The model under review builds one solid part; all positions refer to its coordinate system, in mm. A direction names the side the tool comes from. Coordinates: 2 decimals unless noted, no trailing zeros. Order: outer loops, then holes, each group sorted by start corner. A loop starts at its lowest first (then second) coordinate and runs counter-clockwise, first axis right, second up. Notation, with made-up numbers: M 54.5,-33.5 L 70.5,-33.5 A34 ccw 70.5,-3.5 Z; hole C 44,44 d7. An arc over 180 degrees is marked long. Answer as CSV lines item,"result". Start each with the question number.
Q1. Consider section C-C on x = 0. Write out the cut boundary in (y, z).
Q2. Consider section A-A on z = 0. Write out the cut boundary in (x, y), and give its area (3 significant figures).
Q3. For P1, Ø6.5, axis at x = 30, z = -12.5, coming from the +Y side; P2, Ø6, axis at y = 1.5, z = 11.5, coming from the +X side; P3, Ø1.5, axis at x = 27.5, y = 5, coming from the -Z side, all flat-tipped, find the tip position at first contact; note any pin that passes through.
Q4. The part is to be moulded in two halves that separate along Y. For faces 5 (the face through (15, 12, 24)), 6 (the face through (8.778, 8.307, 18.025)), 7 (the face through (8.69, 10.02, -15.19)), say which applies: +Y half, -Y half, draft (parallel to the pull), parting line (faces both ways), or undercut.
Q5. Machinability: for faces 1 (the face through (27.22, 3.43, -4.4)), 2 (the face through (11.405, 5.555, -14.914)), 3 (the face through (19.769, 9.465, 19.754)), 4 (the face through (-25, 2, -16)), which of the approach directions +Z, -Z, +X, -X, +Y, -Y give a long, thin tool a straight path to every point of the face, cutting with its end or side? Answer none if there is none.
Q6. Consider section B-B on y = 10.75. Write out the cut boundary in (x, z), and give its area (3 significant figures).
Q7. Consider section D-D on x = 31. Write out the cut boundary in (y, z), and give its area (3 significant figures).
Q8. Wall thickness on L1, parallel to X at y = 3.5, z = -13.75; L2, parallel to Z at x = 0, y = 3.7; L3, parallel to Z at x = 0, y = 1.35: over which ranges is each line inside the solid? List them lowest first. Write a range as [from, to].
from build123d import *

# Parameters (mm, degrees)
SKETCH1_R                = 37.5
SKETCH1_R_2              = 2.3
BOSS_EXTRUDE1_DEPTH      = 2
SKETCH2_R                = 37.5
SKETCH2_R_2              = 4.5
BOSS_EXTRUDE2_DEPTH      = 5
BOSS_EXTRUDE3_DEPTH      = 5
SKETCH4_R                = 17.5
CUT_EXTRUDE1_DEPTH       = 7
CUT_EXTRUDE2_DEPTH       = 7
CUT_EXTRUDE2_DEPTH_BACK  = 2.5
CUT_EXTRUDE4_DEPTH       = 3
CUT_EXTRUDE4_DEPTH_BACK  = 2.5
SKETCH10_R               = 1.65
CUT_EXTRUDE7_DEPTH       = 20
SKETCH9_R                = 1.65
CUT_EXTRUDE6_DEPTH       = 20
CUT_EXTRUDE8_DEPTH       = 4
CUT_EXTRUDE9_DEPTH       = 10
CUT_EXTRUDE9_DEPTH_BACK  = 2.5
SKETCH16_R               = 1.65
CUT_EXTRUDE10_DEPTH      = 20
CUT_EXTRUDE11_DEPTH      = 10
CUT_EXTRUDE11_DEPTH_BACK = 2.5
SKETCH18_R               = 1.65
CUT_EXTRUDE12_DEPTH      = 20
FILLET1_R                = 2


with BuildPart() as part:
    # Sketch1 → Boss-Extrude1 (new body)
    with BuildSketch(Plane(origin=(0, 0, 0), x_dir=(1, 0, 0), z_dir=(0, 1, 0))):
        Circle(SKETCH1_R)
        with Locations((0, 27.5)):
            Circle(SKETCH1_R_2, mode=Mode.SUBTRACT)
        with Locations((23.815698604, 13.75)):
            Circle(SKETCH1_R_2, mode=Mode.SUBTRACT)
        with Locations((23.815698604, -13.75)):
            Circle(SKETCH1_R_2, mode=Mode.SUBTRACT)
        with Locations((0, -27.5)):
            Circle(SKETCH1_R_2, mode=Mode.SUBTRACT)
        with Locations((-23.815698604, -13.75)):
            Circle(SKETCH1_R_2, mode=Mode.SUBTRACT)
        with Locations((-23.815698604, 13.75)):
            Circle(SKETCH1_R_2, mode=Mode.SUBTRACT)
    extrude(amount=BOSS_EXTRUDE1_DEPTH)

    # Sketch2 → Boss-Extrude2 (add)
    with BuildSketch(Plane(origin=(0, 2, 0), x_dir=(1, 0, 0), z_dir=(0, 1, 0))):
        Circle(SKETCH2_R)
        with Locations((-23.815698604, 13.75)):
            Circle(SKETCH2_R_2, mode=Mode.SUBTRACT)
        with Locations((-23.815698604, -13.75)):
            Circle(SKETCH2_R_2, mode=Mode.SUBTRACT)
        with Locations((0, -27.5)):
            Circle(SKETCH2_R_2, mode=Mode.SUBTRACT)
        with Locations((23.815698604, -13.75)):
            Circle(SKETCH2_R_2, mode=Mode.SUBTRACT)
        with Locations((23.815698604, 13.75)):
            Circle(SKETCH2_R_2, mode=Mode.SUBTRACT)
        with Locations((0, 27.5)):
            Circle(SKETCH2_R_2, mode=Mode.SUBTRACT)
    extrude(amount=BOSS_EXTRUDE2_DEPTH)

    # Sketch3 → Boss-Extrude3 (add)
    with BuildSketch(Plane(origin=(0, 7, 0), x_dir=(1, 0, 0), z_dir=(0, 1, 0))):
        with BuildLine():
            ThreePointArc((-16.901898546, -4.536058371), (-17.499998615, -0.006962688), (-16.905502698, 4.52260749))
            Line((-16.905502698, 4.52260749), (-36.226077211, 9.691301765))
            ThreePointArc((-36.226077211, 9.691301765), (-37.499997032, -0.014920046), (-36.218354027, -9.720125081))
            Line((-36.218354027, -9.720125081), (-16.901898546, -4.536058371))
        make_face()
        with BuildLine():
            ThreePointArc((-9.720125081, 36.218354027), (-18.762919655, 32.468490048), (-26.527052262, 26.50595213))
            Line((-26.527052262, 26.50595213), (-12.810223172, 12.800033673))
            Line((-12.810223172, 12.800033673), (-4.698199739, 17.506056765))
            Line((-4.698199739, 17.506056765), (-9.720125081, 36.218354027))
        make_face()
        with BuildLine():
            ThreePointArc((16.901898546, 4.536058371), (17.499998615, 0.006962688), (16.905502698, -4.52260749))
            Line((16.905502698, -4.52260749), (36.226077211, -9.691301765))
            ThreePointArc((36.226077211, -9.691301765), (37.499997032, 0.014920046), (36.218354027, 9.720125081))
            Line((36.218354027, 9.720125081), (16.901898546, 4.536058371))
        make_face()
        with BuildLine():
            Line((-12.805791077, -12.81598516), (-26.50595213, -26.527052262))
            ThreePointArc((-26.50595213, -26.527052262), (-18.737077377, -32.483410095), (-9.691301765, -36.226077211))
            Line((-9.691301765, -36.226077211), (-4.682147808, -17.501864262))
            Line((-4.682147808, -17.501864262), (-12.805791077, -12.81598516))
        make_face()
        with BuildLine():
            Line((4.680172315, 17.49447987), (12.811230656, 12.82142907))
            Line((12.811230656, 12.82142907), (26.50595213, 26.527052262))
            ThreePointArc((26.50595213, 26.527052262), (18.737077377, 32.483410095), (9.691301765, 36.226077211))
            Line((9.691301765, 36.226077211), (4.680172315, 17.49447987))
        make_face()
        with BuildLine():
            Line((12.819708432, -12.809511387), (4.694715176, -17.493072864))
            Line((4.694715176, -17.493072864), (9.720125081, -36.218354027))
            ThreePointArc((9.720125081, -36.218354027), (18.762919655, -32.468490048), (26.527052262, -26.50595213))
            Line((26.527052262, -26.50595213), (12.819708432, -12.809511387))
        make_face()
    extrude(amount=BOSS_EXTRUDE3_DEPTH)

    # Sketch4 → Cut-Extrude1 (cut)
    with BuildSketch(Plane(origin=(0, 7, 0), x_dir=(1, 0, 0), z_dir=(0, 1, 0))):
        Circle(SKETCH4_R)
    extrude(amount=-CUT_EXTRUDE1_DEPTH, mode=Mode.SUBTRACT)

    # Sketch5 → Cut-Extrude2 (cut, two sides)
    with BuildSketch(Plane(origin=(-8.743969443, 0, 15.158924711), x_dir=(-0.866224269, 0, -0.499655397), z_dir=(0.499655397, 0, -0.866224269))) as cut_extrude2_sk:
        with BuildLine():
            Line((1.5, 7), (3.290896534, 7))
            Line((3.290896534, 7), (1.645448267, 9.85))
            Line((1.645448267, 9.85), (-1.645448267, 9.85))
            Line((-1.645448267, 9.85), (-3.290896534, 7))
            Line((-3.290896534, 7), (-1.5, 7))
            ThreePointArc((-1.5, 7), (0, 8.5), (1.5, 7))
        make_face()
        with BuildLine():
            Line((1.645448267, 4.15), (3.290896534, 7))
            Line((3.290896534, 7), (1.5, 7))
            ThreePointArc((1.5, 7), (0, 5.5), (-1.5, 7))
            Line((-1.5, 7), (-3.290896534, 7))
            Line((-3.290896534, 7), (-1.645448267, 4.15))
            Line((-1.645448267, 4.15), (1.645448267, 4.15))
        make_face()
        with BuildLine():
            ThreePointArc((-1.5, 7), (0, 5.5), (1.5, 7))
            Line((1.5, 7), (0, 7))
            Line((0, 7), (-1.5, 7))
        make_face()
        with BuildLine():
            Line((0, 7), (1.5, 7))
            ThreePointArc((1.5, 7), (0, 8.5), (-1.5, 7))
            Line((-1.5, 7), (0, 7))
        make_face()
    extrude(amount=CUT_EXTRUDE2_DEPTH, mode=Mode.SUBTRACT)
    extrude(cut_extrude2_sk.sketch, amount=-CUT_EXTRUDE2_DEPTH_BACK, mode=Mode.SUBTRACT)

    # Sketch7 → Cut-Extrude4 (cut, two sides)
    with BuildSketch(Plane(origin=(8.739633736, 0, 15.161424807), x_dir=(-0.866367132, 0, 0.499407642), z_dir=(-0.499407642, 0, -0.866367132))) as cut_extrude4_sk:
        Polygon((0, 7), (3.270607136, 7), (1.625158868, 9.85), (-1.665737666, 9.85), (-3.311185933, 7), (-0.020289399, 7), align=None)
        Polygon((1.625158868, 4.15), (3.270607136, 7), (0, 7), (-0.020289399, 7), (-3.311185933, 7), (-1.665737666, 4.15), align=None)
    extrude(amount=CUT_EXTRUDE4_DEPTH, mode=Mode.SUBTRACT)
    extrude(cut_extrude4_sk.sketch, amount=-CUT_EXTRUDE4_DEPTH_BACK, mode=Mode.SUBTRACT)

    # Sketch10 → Cut-Extrude7 (cut)
    with BuildSketch(Plane(origin=(8.739633736, 0, 15.161424807), x_dir=(-0.866367132, 0, 0.499407642), z_dir=(-0.499407642, 0, -0.866367132))):
        with Locations((-0.020289399, 7)):
            Circle(SKETCH10_R)
    extrude(amount=-CUT_EXTRUDE7_DEPTH, mode=Mode.SUBTRACT)

    # Sketch9 → Cut-Extrude6 (cut)
    with BuildSketch(Plane(origin=(-9.993107934, 0, 17.324485384), x_dir=(-0.866224269, 0, -0.499655397), z_dir=(0.499655397, 0, -0.866224269))):
        with Locations((0, 6.9)):
            Circle(SKETCH9_R)
    extrude(amount=-CUT_EXTRUDE6_DEPTH, mode=Mode.SUBTRACT)

    # Sketch14 → Cut-Extrude8 (cut)
    with BuildSketch(Plane.XZ):
        with BuildLine():
            Line((17.5, 0), (37.5, 0))
            ThreePointArc((37.5, 0), (37.416199333, 2.505599224), (37.165171868, 5))
            Line((37.165171868, 5), (16.770509831, 5))
            ThreePointArc((16.770509831, 5), (17.316667145, 2.526467688), (17.5, 0))
        make_face()
        with BuildLine():
            Line((16.770509831, -5), (37.165171868, -5))
            ThreePointArc((37.165171868, -5), (37.416199333, -2.505599224), (37.5, 0))
            Line((37.5, 0), (17.5, 0))
            ThreePointArc((17.5, 0), (17.316667145, -2.526467688), (16.770509831, -5))
        make_face()
    extrude(amount=-CUT_EXTRUDE8_DEPTH, mode=Mode.SUBTRACT)

    # Sketch15 → Cut-Extrude9 (cut, two sides)
    with BuildSketch(Plane(origin=(-8.781531952, 0, -15.137195796), x_dir=(0.864982617, 0, -0.501801826), z_dir=(0.501801826, 0, 0.864982617))) as cut_extrude9_sk:
        with BuildLine():
            Line((0, 7), (1.5, 7))
            ThreePointArc((1.5, 7), (0, 8.5), (-1.5, 7))
            Line((-1.5, 7), (0, 7))
        make_face()
        with BuildLine():
            ThreePointArc((-1.5, 7), (0, 5.5), (1.5, 7))
            Line((1.5, 7), (0, 7))
            Line((0, 7), (-1.5, 7))
        make_face()
        with BuildLine():
            Line((1.645448267, 4.15), (3.290896534, 7))
            Line((3.290896534, 7), (1.5, 7))
            ThreePointArc((1.5, 7), (0, 5.5), (-1.5, 7))
            Line((-1.5, 7), (-3.290896534, 7))
            Line((-3.290896534, 7), (-1.645448267, 4.15))
            Line((-1.645448267, 4.15), (1.645448267, 4.15))
        make_face()
        with BuildLine():
            Line((1.5, 7), (3.290896534, 7))
            Line((3.290896534, 7), (1.645448267, 9.85))
            Line((1.645448267, 9.85), (-1.645448267, 9.85))
            Line((-1.645448267, 9.85), (-3.290896534, 7))
            Line((-3.290896534, 7), (-1.5, 7))
            ThreePointArc((-1.5, 7), (0, 8.5), (1.5, 7))
        make_face()
    extrude(amount=CUT_EXTRUDE9_DEPTH, mode=Mode.SUBTRACT)
    extrude(cut_extrude9_sk.sketch, amount=-CUT_EXTRUDE9_DEPTH_BACK, mode=Mode.SUBTRACT)

    # Sketch16 → Cut-Extrude10 (cut)
    with BuildSketch(Plane(origin=(-10.036036516, 0, -17.299652339), x_dir=(0.864982617, 0, -0.501801826), z_dir=(0.501801826, 0, 0.864982617))):
        with Locations((0, 7)):
            Circle(SKETCH16_R)
    extrude(amount=-CUT_EXTRUDE10_DEPTH, mode=Mode.SUBTRACT)

    # Sketch17 → Cut-Extrude11 (cut, two sides)
    with BuildSketch(Plane(origin=(8.720008177, 0, -15.17272083), x_dir=(0.867012619, 0, 0.498286182), z_dir=(-0.498286182, 0, 0.867012619))) as cut_extrude11_sk:
        Polygon((3.290896534, 7), (1.645448267, 9.85), (-1.645448267, 9.85), (-3.290896534, 7), (-1.645448267, 4.15), (1.645448267, 4.15), align=None)
    extrude(amount=CUT_EXTRUDE11_DEPTH, mode=Mode.SUBTRACT)
    extrude(cut_extrude11_sk.sketch, amount=-CUT_EXTRUDE11_DEPTH_BACK, mode=Mode.SUBTRACT)

    # Sketch18 → Cut-Extrude12 (cut)
    with BuildSketch(Plane(origin=(9.965723631, 0, -17.340252378), x_dir=(0.867012619, 0, 0.498286182), z_dir=(-0.498286182, 0, 0.867012619))):
        with Locations((0, 7)):
            Circle(SKETCH18_R)
    extrude(amount=-CUT_EXTRUDE12_DEPTH, mode=Mode.SUBTRACT)

    # Fillet1
    fillet1_edges = [part.edges().sort_by_distance(p)[0] for p in [
        (26.96784085, 4, 5),
        (26.96784085, 4, -5),
    ]]
    fillet(fillet1_edges, radius=FILLET1_R)


solid = part.part
Evaluation:
1,outline,"M 0,-37.5 L 7,-37.5 L 7,-32 L 2,-32 L 2,-29.8 L 0,-29.8 Z; M 0,-25.2 L 2,-25.2 L 2,-23 L 7,-23 L 7,-17.5 L 0,-17.5 Z; M 0,17.5 L 7,17.5 L 7,23 L 2,23 L 2,25.2 L 0,25.2 Z; M 0,29.8 L 2,29.8 L 2,32 L 7,32 L 7,37.5 L 0,37.5 Z"
2,outline,"M -37.5,0 L -17.5,0 L -17.5,12 L -37.5,12 Z; M 17.5,4 L 37.5,4 L 37.5,12 L 17.5,12 Z"
2,area,"400 mm²"
3,P1,"stops at y = 7"
3,P2,"stops at x = 36.52"
3,P3,"stops at z = -26.28"
4,face 5,"+Y half"
4,face 6,"undercut"
4,face 7,"draft"
5,face 1,"+X, -Y"
5,face 2,"none"
5,face 3,"+X, +Y"
5,face 4,"+Y"
6,outline,"M -36.23,-9.69 L -16.91,-4.52 A17.5 cw -16.9,4.54 L -36.22,9.72 A37.5 ccw Z; M -26.53,-26.51 A37.5 ccw -9.72,-36.22 L -4.7,-17.51 L -12.81,-12.8 Z; M -26.51,26.53 L -12.81,12.82 L -4.68,17.5 L -9.69,36.23 A37.5 ccw Z; M 4.68,-17.49 L 9.69,-36.23 A37.5 ccw 26.51,-26.53 L 12.81,-12.82 Z; M 4.69,17.49 L 12.82,12.81 L 26.53,26.51 A37.5 ccw 9.72,36.22 Z; M 16.9,-4.54 L 36.22,-9.72 A37.5 ccw 36.23,9.69 L 16.91,4.52 A17.5 cw Z"
6,area,"1,720 mm²"
7,outline,"M 0,-21.1 L 7,-21.1 L 7,-8.32 L 12,-8.32 L 12,8.29 L 7,8.29 L 7,21.1 L 0,21.1 L 0,5 L 2,5 A2 cw 4,3 L 4,-3 A2 cw 2,-5 L 0,-5 Z"
7,area,"340 mm²"
8,L1,"x = [-34.89, -28.32], [-19.32, -10.83], [10.83, 19.32], [28.32, 34.89]"
8,L2,"z = [-37.5, -32], [-23, -17.5], [17.5, 23], [32, 37.5]"
8,L3,"z = [-37.5, -29.8], [-25.2, -17.5], [17.5, 25.2], [29.8, 37.5]"
